Could you check a few things on this model? Use its own coordinates, in mm. A direction names the side the tool comes from. Coordinates: 2 decimals unless noted, no trailing zeros. Write each loop counter-clockwise with the first axis right and the second up, starting at its lowest first coordinate (ties: lowest second). Pieces come first, ordered by that corner, then holes.
```python
from build123d import *

# Parameters (mm, degrees)
SALIENTE_EXTRUIR1_DEPTH = 11
CROQUIS2_R              = 1.45
CORTAR_EXTRUIR1_DEPTH   = 11
CORTAR_EXTRUIR2_DEPTH   = 7


with BuildPart() as part:
    # Croquis1 → Saliente-Extruir1 (new body)
    with BuildSketch(Plane(origin=(0, -33.400588291, 0), x_dir=(1, 0, 0), z_dir=(0, 1, 0))):
        with BuildLine():
            Line((-45.256444502, -97.372583002), (-33.235629222, -109.393398282))
            ThreePointArc((-33.235629222, -109.393398282), (-26.16456141, -109.393398282), (-26.16456141, -102.32233047))
            Line((-26.16456141, -102.32233047), (-38.18537669, -90.30151519))
            ThreePointArc((-38.18537669, -90.30151519), (-45.256444502, -90.30151519), (-45.256444502, -97.372583002))
        make_face()
    extrude(amount=SALIENTE_EXTRUIR1_DEPTH)

    # Croquis2 → Cortar-Extruir1 (cut)
    with BuildSketch(Plane.XZ.offset(33.400588291)):
        with Locations((-41.720910596, 93.837049096)):
            Circle(CROQUIS2_R)
        with Locations((-29.700095316, 105.857864376)):
            Circle(CROQUIS2_R)
    extrude(amount=-CORTAR_EXTRUIR1_DEPTH, mode=Mode.SUBTRACT)

    # Croquis3 → Cortar-Extruir2 (cut)
    with BuildSketch(Plane.XZ.offset(33.400588291)):
        Polygon((-40.24952431, 104.38647809), (-37.421097185, 107.214905215), (-26.82292811, 96.61673614), (-32.47978236, 90.95988189), (-43.077951435, 101.558050965), align=None)
    extrude(amount=-CORTAR_EXTRUIR2_DEPTH, mode=Mode.SUBTRACT)


solid = part.part
```
1. I want a section at D-D on z = 99.5. Please give me the cut outline in (x, y), plus the area to 3 significant figures.
Verdict:
outline: (-43.13, -33.4) - (-41.02, -33.4) - (-41.02, -26.4) - (-29.71, -26.4) - (-29.71, -33.4) - (-28.99, -33.4) - (-28.99, -22.4) - (-43.13, -22.4) - close
area: 76.4 mm2
2. I want a section at A-A on z = 94.5. Please give me the cut outline in (x, y), plus the area to 3 significant figures.
Verdict:
outline: (-46.68, -33.4) - (-43.01, -33.4) - (-43.01, -22.4) - (-46.68, -22.4) - close; (-40.43, -33.4) - (-36.02, -33.4) - (-36.02, -26.4) - (-33.99, -26.4) - (-33.99, -22.4) - (-40.43, -22.4) - close
area: 97.0 mm2
3. If we mould it in two halves opening along Z, with no side actions, what happens to faces 1 (the face through (-36, -22.401, 100)), 2 (the face through (-42.79, -27.978, 94.817)), 3 (the face through (-26.24, -27.98, 109.47))? For each: pulls with the +Z half, pulls with the -Z half, needs draft (parallel to the pull), parting line crosses it, or undercut.
Verdict:
face 1: needs draft
face 2: undercut
face 3: parting line crosses it
4. I want a section at B-B on y = -32.25. Please give me the cut outline in (x, z), plus the area to 3 significant figures.
Verdict:
outline: (-45.26, 97.37) arc R5 ccw to (-38.19, 90.3) - (-35, 93.48) - (-42.07, 100.55) - close; (-36.42, 106.21) - (-29.35, 99.14) - (-26.16, 102.32) arc R5 ccw to (-33.24, 109.39) - close; hole circle Ø2.9 at (-41.72, 93.84); hole circle Ø2.9 at (-29.7, 105.86)
area: 155 mm2
5. For pin 1 (2 mm diameter, centred on x = -36.5, y = -26, fed in from +Z); pin 2 (6 mm diameter, centred on x = -38.5, y = -29.5, fed in from -Z); pin 3 (1.5 mm diameter, centred on x = -32, y = -28, fed in from -Z), each with a flat end and sliding along its axis, tell me the tip position at first contact or that it passes through.
Verdict:
pin 1: stops at z = 107.13
pin 2: stops at z = 88.84
pin 3: stops at z = 101.04
6. I want a section at C-C on x = -30. Please give me the cut outline in (y, z).
Verdict:
outline: (-33.4, 99.79) - (-26.4, 99.79) - (-26.4, 98.49) - (-22.4, 98.49) - (-22.4, 104.44) - (-33.4, 104.44) - close; (-33.4, 107.28) - (-22.4, 107.28) - (-22.4, 110.85) - (-33.4, 110.85) - close
7. On a 3-axis mill with a long thin cutter (end or side, diameter ignored), from which of +Z, -Z, +X, -X, +Y, -Y can I reach the whole of each face in a straight line? I mean faces 4 (the face through (-36, -26.401, 100)), 5 (the face through (-39.33, -25.53, 103.3)). Say none if no direction works.
Verdict:
face 4: -Y
face 5: +Z, -X, +Y, -Y
8. Please list where these lines run through material, in increasing order: line 1 along Y through (x, z) = (-36, 97.5); line 2 along X through (y, z) = (-23, 106.25); line 3 along Z through (x, y) = (-29.5, -33).
Verdict:
line 1: y = -26.4 to -22.4
line 2: x = -36.38 to -31.1, -28.3 to -24.72
line 3: z = 99.29 to 104.42, 107.29 to 110.85
